Could you check a few things on this model? Use its own coordinates, in mm. Round coordinates to 2 decimals unless told otherwise and drop trailing zeros. Loops run counter-clockwise (first coordinate to the right, second up) from the corner with the lowest first, then second, coordinate; pieces in that order, holes last. Notation, with made-up numbers: (18, 89.25) -> (54, 89.25) arc R17 ccw to (54, 105.25) -> close; hole circle Ø7 at (-20, 5.25). An arc over 180 degrees is marked (long way). One line per item, written item: value.
```python
from build123d import *

# Parameters (mm, degrees)
F0_W     = 12
F0_H     = 28
F0_R     = 1.5
F1_DEPTH = 8
F2_R     = 1


with BuildPart() as f1:
    # F0 (on Top) → F1 (new body)
    with BuildSketch(Plane.XY):
        Rectangle(F0_W, F0_H)
        with Locations((0, 11.324412)):
            Circle(F0_R, mode=Mode.SUBTRACT)
    extrude(amount=F1_DEPTH)

    # F2
    f2_edges = [f1.edges().sort_by_distance(p)[0] for p in [
        (0, 14, 8),
        (6, 0, 8),
        (-6, 0, 8),
        (0, -14, 8),
        (6, 14, 4),
        (-6, 14, 4),
        (0, 14, 0),
        (6, 0, 0),
        (-6, 0, 0),
        (0, -14, 0),
        (6, -14, 4),
        (-6, -14, 4),
    ]]
    fillet(f2_edges, radius=F2_R)


solid = f1.part
```
Item 1: I need wall thicknesses on line 1 (Y direction, x = 0, z = 5.75); line 2 (X direction, y = 11, z = 1.5); line 3 (Y direction, x = 1.25, z = 7). Which ranges of each line are inside material? Lowest first, please. Write a range as from..to.
Output:
line 1: y = -14..9.82, 12.82..14
line 2: x = -6..-1.46, 1.46..6
line 3: y = -14..10.5, 12.15..14
Item 2: If we section it at A-A on x = 0: List the corners of the cut face in (y, z) for me.
Output:
outline: (-14, 1) arc R1 ccw to (-13, 0) -> (9.82, 0) -> (9.82, 8) -> (-13, 8) arc R1 ccw to (-14, 7) -> close; (12.82, 0) -> (13, 0) arc R1 ccw to (14, 1) -> (14, 7) arc R1 ccw to (13, 8) -> (12.82, 8) -> close
Item 3: If we mould it in two halves opening along Y, with no side actions, what happens to faces 1 (the face through (-0.33, 9.86, 3.94)), 2 (the face through (0.07, -13.715, 0.301)), 3 (the face through (0.07, 13.715, 0.301)), 4 (the face through (-6, 0, 4))? For each: released by +Y, released by -Y, zero draft, split by the parting line, or undercut.
Output:
face 1: undercut
face 2: released by -Y
face 3: released by +Y
face 4: zero draft
Item 4: Will this pin go through, and if not, where does the flat tip stop? pin 1 Ø1.8 at (x, y) = (0, 11.32) entering from -Z (3 decimals).
Output:
pin 1: passes through
Item 5: If we section it at B-B on z = 4.5: List the corners of the cut face in (x, y) for me.
Output:
outline: (-6, -13) arc R1 ccw to (-5, -14) -> (5, -14) arc R1 ccw to (6, -13) -> (6, 13) arc R1 ccw to (5, 14) -> (-5, 14) arc R1 ccw to (-6, 13) -> close; hole circle Ø3 at (0, 11.32)
